Input: dimensioned drawing with shaded views. Units: mm. Origin: part minimum x, y, z. A direction names the side the tool comes from. Round coordinates to 2 decimals unless told otherwise and drop trailing zeros. Loops run counter-clockwise (first coordinate to the right, second up) from the corner with the lowest first, then second, coordinate; pieces in that order, holes last. Notation, with made-up numbers: (62.25, -40) - (99.25, -40) arc R24 cw to (99.25, -24) - close; hole circle Ø6 at (39.5, -39). An arc over 180 degrees is marked (long way). Answer as CSV lines item,"result".
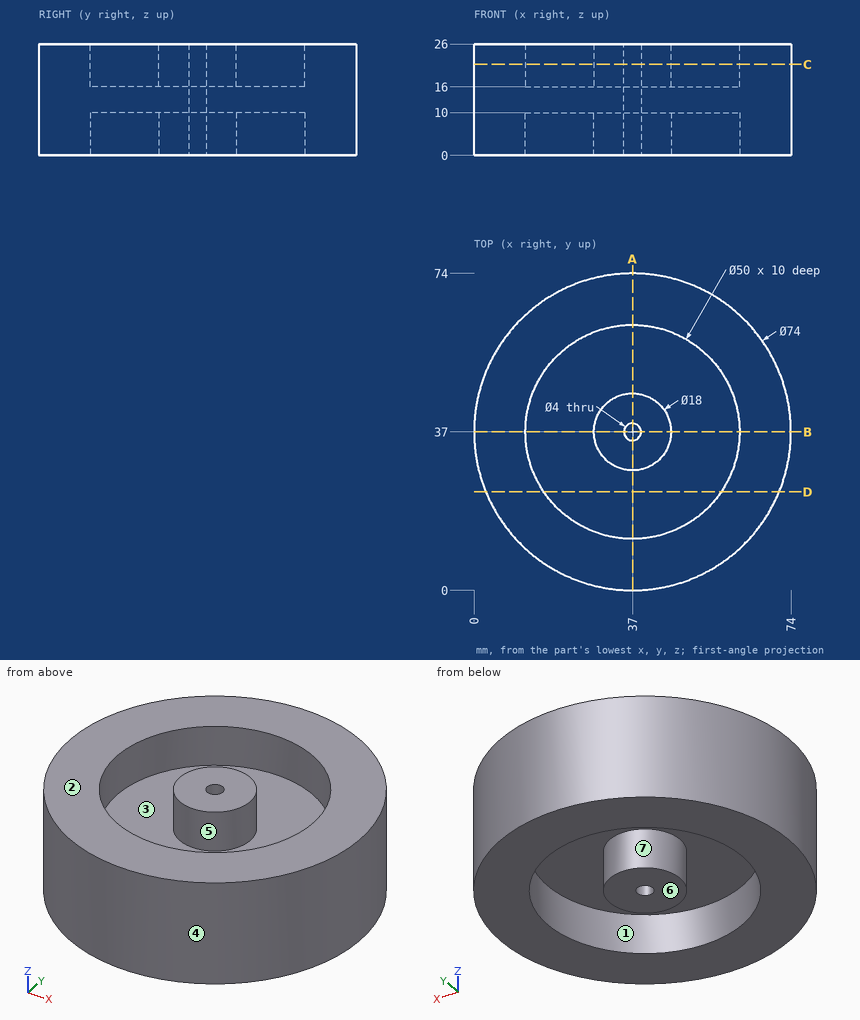
(1) Pin query (flat end, axial travel): P1, Ø1, axis at y = 20, z = 9, coming from the +X side; P2, Ø1.5, axis at x = 65, z = 21, coming from the -Y side; P3, Ø12, axis at x = 27, z = 13, coming from the +Y side. Return the tip coordinate at first contact, or that it passes through.
Findings below:
P1,"x = 70.12"
P2,"y = 11.97"
P3,"y = 73.78"
(2) Section C-C (z = 21.25). Output: boundary loops of the cut face in (x, y).
Findings below:
outline,"circle Ø74 at (37, 37); circle Ø18 at (37, 37); hole circle Ø50 at (37, 37); hole circle Ø4 at (37, 37)"
(3) Section D-D (y = 23). Output: boundary loops of the cut face in (x, z).
Findings below:
outline,"(2.75, 0) - (16.29, 0) - (16.29, 10) - (57.71, 10) - (57.71, 0) - (71.25, 0) - (71.25, 26) - (57.71, 26) - (57.71, 16) - (16.29, 16) - (16.29, 26) - (2.75, 26) - close"
(4) Section A-A (x = 37). Output: boundary loops of the cut face in (y, z).
Findings below:
outline,"(0, 0) - (12, 0) - (12, 10) - (28, 10) - (28, 0) - (35, 0) - (35, 26) - (28, 26) - (28, 16) - (12, 16) - (12, 26) - (0, 26) - close; (39, 0) - (46, 0) - (46, 10) - (62, 10) - (62, 0) - (74, 0) - (74, 26) - (62, 26) - (62, 16) - (46, 16) - (46, 26) - (39, 26) - close"
(5) Access query for the marked faces 1, 2 and 3. Directions: +Z, -Z, +X, -X, +Y, -Y. A direction counts if a zero-diameter tool reaches every point of the face in a straight line with its end or side. Return the directions, or none.
Findings below:
face 1,"-Z"
face 2,"+Z, +X, -X, +Y, -Y"
face 3,"+Z"
(6) Material intervals for line 1 along Y through (x, z) = (37, 4.25); line 2 along Y through (x, z) = (40, 21); line 3 along Y through (x, z) = (43.5, 5), sorted ascending.
Findings below:
line 1,"0 to 12, 28 to 35, 39 to 46, 62 to 74"
line 2,"0.12 to 12.18, 28.51 to 45.49, 61.82 to 73.88"
line 3,"0.58 to 12.86, 30.78 to 43.22, 61.14 to 73.42"
(7) Draft query along X for the marked faces 4, 5, 6 and 7. Return one class per face: pulls with the +X half, pulls with the -X half, needs draft (parallel to the pull), parting line crosses it, or undercut.
Findings below:
face 4,"parting line crosses it"
face 5,"undercut"
face 6,"needs draft"
face 7,"undercut"
